Check sheet for the drawn part. Datum: minimum x, y, z corner. Units: mm. Round coordinates to 2 decimals unless told otherwise and drop trailing zeros. Write each loop counter-clockwise with the first axis right and the second up, starting at its lowest first coordinate (ties: lowest second). Pieces come first, ordered by that corner, then holes. Notation, with made-up numbers: M -21.75,18 L 18.25,18 A8 ccw 18.25,27 Z; hole C 32,65.25 d3. An arc over 180 degrees is marked long. One line per item, written item: value. Start each with the question number.
Item 1: Thickness scan on probe 1 along X at (y, z) = (2.4, 106); probe 2 along Z at (x, y) = (60, 2.35) (3 decimals). Record the ranges inside material, lowest first. Write a range as from..to.
Item 2: Gauge pin test, flat ends, axial feed: pin 1 (1 mm diameter, centred on y = 1, z = 93, fed in from +X); pin 2 (1 mm diameter, centred on y = 2, z = 132.5, fed in from +X); pin 3 (1.6 mm diameter, centred on y = 1.5, z = 132.5, fed in from -X). Record the tip position at first contact, or that the pin passes through.
Item 3: Section check A-A, the plane y = 2.4. Record the cut outline in (x, z) (3 decimals).
Item 4: Section check C-C, the plane x = 49. Record the cut outline in (y, z) (3 decimals), then the cut area to 3 significant figures.
Item 5: Section check B-B, the plane z = 9.5. Record the cut outline in (x, y) (3 decimals).
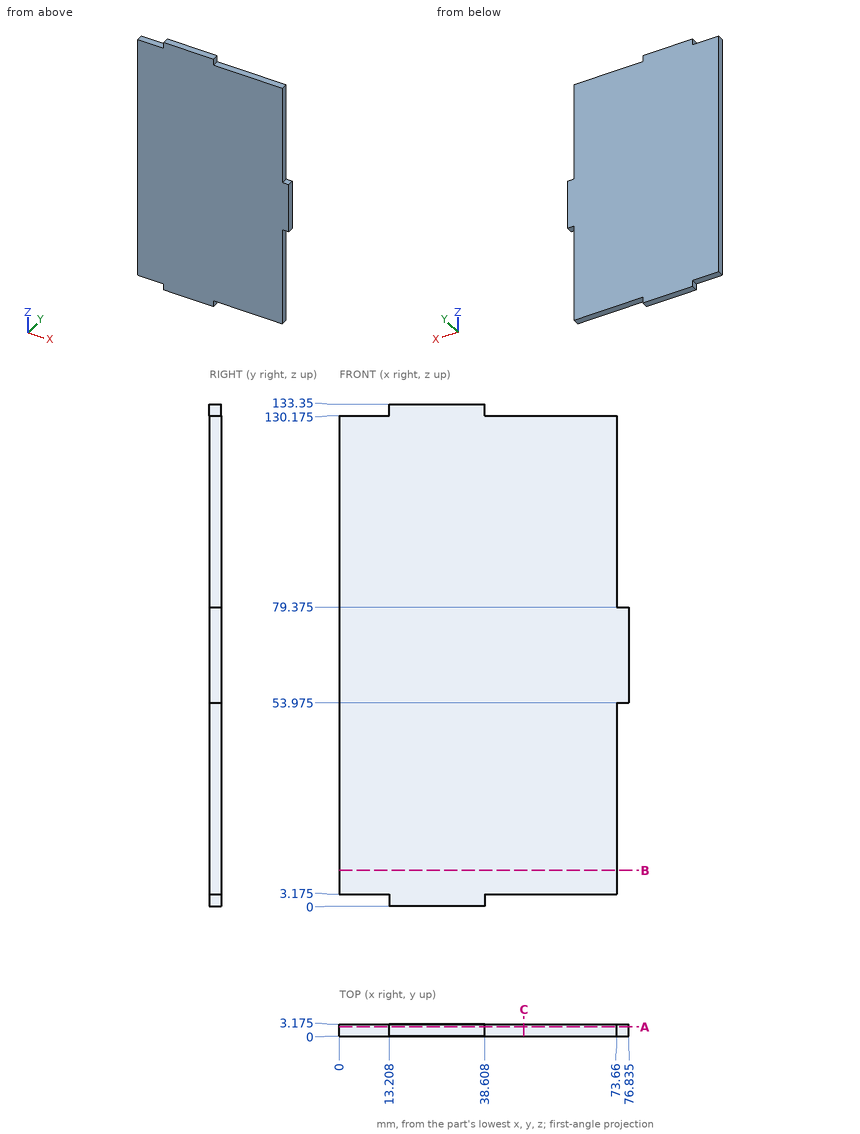
Response values:
1. probe 1: x = 0..73.66
1. probe 2: z = 3.175..130.175
2. pin 1: stops at x = 73.66
2. pin 2: stops at x = 38.61
2. pin 3: stops at x = 13.21
3. outline: M 0,3.175 L 13.208,3.175 L 13.208,0 L 38.608,0 L 38.608,3.175 L 73.66,3.175 L 73.66,53.975 L 76.835,53.975 L 76.835,79.375 L 73.66,79.375 L 73.66,130.175 L 38.608,130.175 L 38.608,133.35 L 13.208,133.35 L 13.208,130.175 L 0,130.175 Z
4. outline: M 0,3.175 L 3.175,3.175 L 3.175,130.175 L 0,130.175 Z
4. area: 403 mm2
5. outline: M 0,0 L 73.66,0 L 73.66,3.175 L 0,3.175 Z
